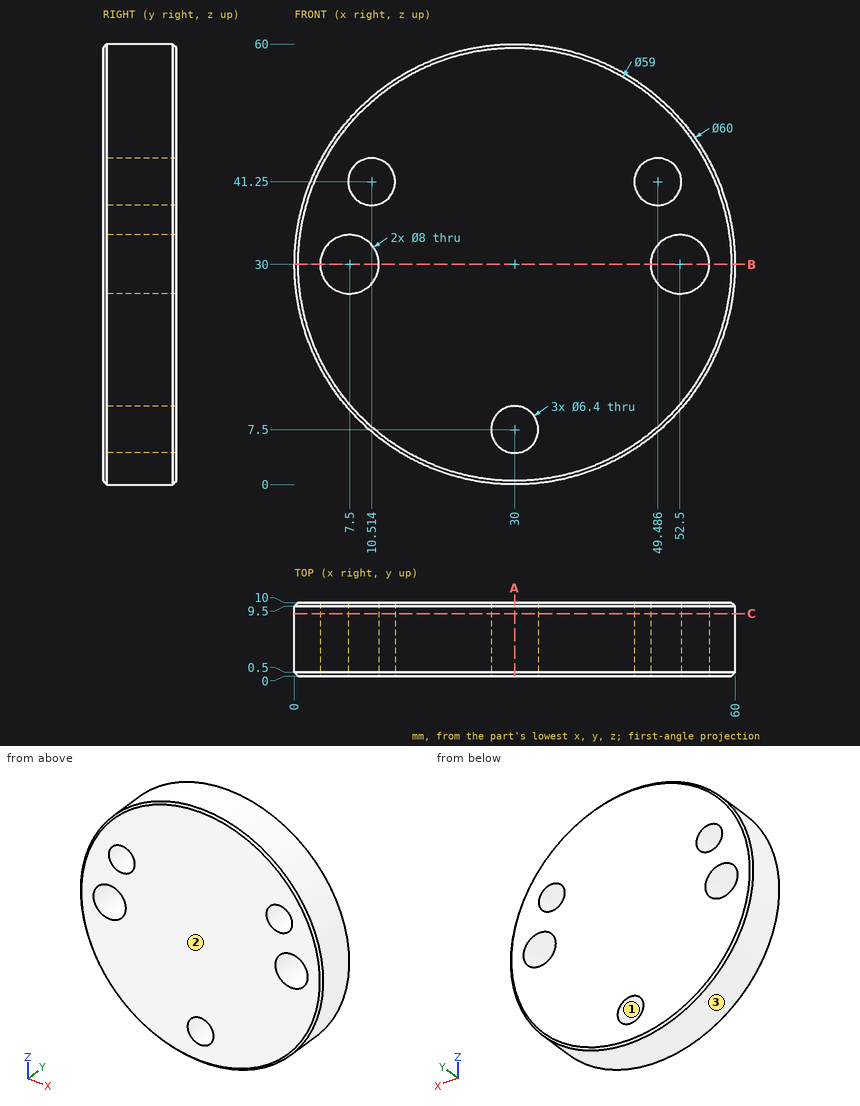
Answer from the drawing. Dimensions are ordinates in mm from the lowest x, y and z of the part. Give positions to 0.01 mm unless a question says otherwise; leave off trailing zeros. Write each loop counter-clockwise with the first axis right and the second up, starting at its lowest first coordinate (ties: lowest second). Pieces come first, ordered by that corner, then holes. Notation, with made-up numbers: (1, 85) - (37, 85) arc R8 cw to (37, 100) - close; hole circle Ø11 at (8.25, 45). An arc over 180 degrees is marked (long way). One line per item, written item: value. Start each with the question number.
1. Given pin 1 (4 mm diameter, centred on x = 30, z = 7.5, fed in from -Y); pin 2 (5 mm diameter, centred on y = 3.5, z = 35, fed in from -X); pin 3 (1 mm diameter, centred on x = 39, y = 5.5, fed in from -Z); pin 4 (4 mm diameter, centred on x = 9.5, y = 5.5, fed in from -Z), each flat-ended and moving along its own axis, determine where each tip first touches the part or whether it passes through.
2. Find section C-C (y = 8.5). State how many separate pieces and enclosed holes the cut face has, then the cut area to 3 significant figures.
3. Find section B-B (z = 30). Write down the section's boundary in (x, y).
4. For a pull along X with two mould halves and no side action, classify the marked faces 1, 2 and 3 as +X half, -X half, draft (parallel to the pull), parting line (faces both ways), or undercut.
5. Consider probe 1 along X at (y, z) = (7.25, 30); probe 2 along X at (y, z) = (3, 39); probe 3 along Z at (x, y) = (49, 2) (1 decimal). Determine where each line is inside the solid, lowest interval first.
6. Find section A-A (x = 30). Write down the section's boundary in (y, z).
Geometry results:
1. pin 1: through
1. pin 2: x = 0.1
1. pin 3: z = 1.23
1. pin 4: z = 6.38
2. separate pieces: 1
2. enclosed holes: 5
2. area: 2,630 mm2
3. outline: (0, 0.5) - (0.5, 0) - (3.5, 0) - (3.5, 10) - (0.5, 10) - (0, 9.5) - close; (11.5, 0) - (48.5, 0) - (48.5, 10) - (11.5, 10) - close; (56.5, 0) - (59.5, 0) - (60, 0.5) - (60, 9.5) - (59.5, 10) - (56.5, 10) - close
4. face 1: undercut
4. face 2: draft
4. face 3: parting line
5. probe 1: 0 to 3.5, 11.5 to 48.5, 56.5 to 60
5. probe 2: 1.38 to 8.24, 12.79 to 47.21, 51.76 to 58.62
5. probe 3: 6.8 to 28.1, 31.9 to 38.1, 44.4 to 53.2
6. outline: (0, 0.5) - (0.5, 0) - (9.5, 0) - (10, 0.5) - (10, 4.3) - (0, 4.3) - close; (0, 10.7) - (10, 10.7) - (10, 59.5) - (9.5, 60) - (0.5, 60) - (0, 59.5) - close
